Check sheet for the drawn part. Datum: minimum x, y, z corner. Units: mm. A direction names the side the tool comes from. Coordinates: 2 decimals unless noted, no trailing zeros. Loops run counter-clockwise (first coordinate to the right, second up) from the corner with the lowest first, then second, coordinate; pieces in that order, holes last.
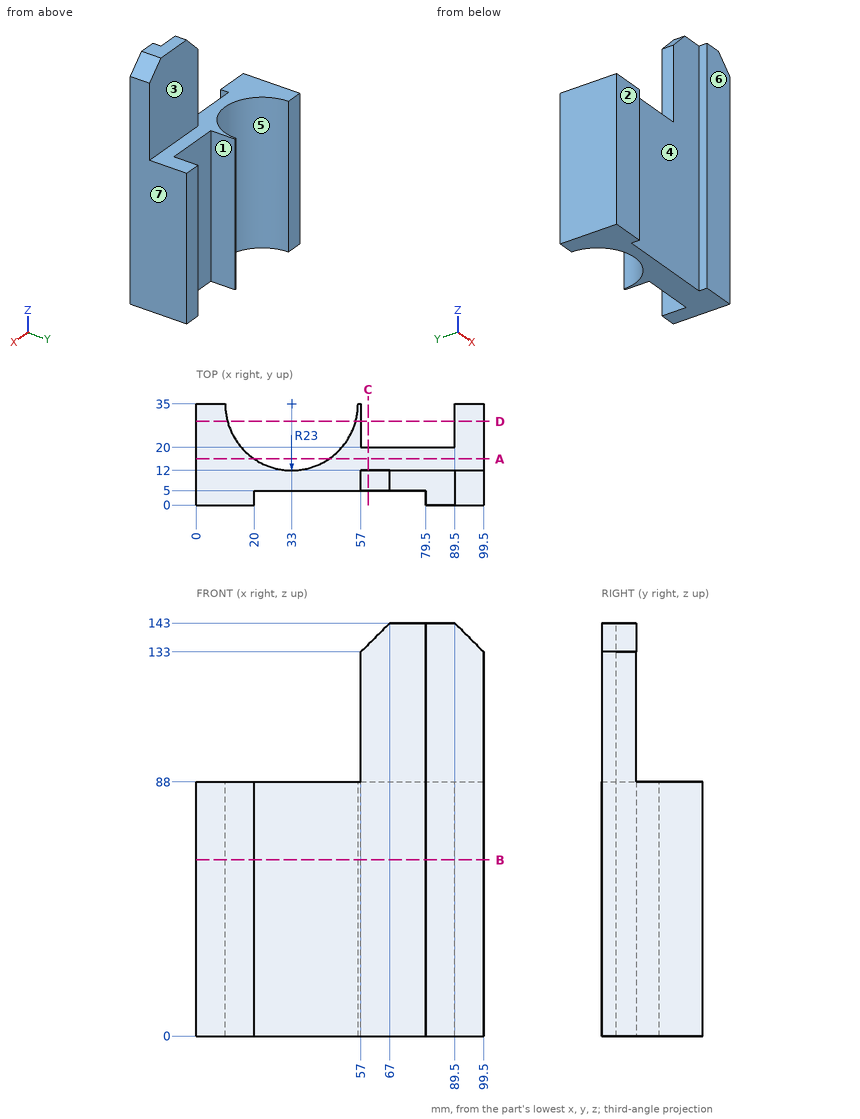
(1) Sectioned sample at A-A on y = 16. Record the cut outline in (x, z).
Findings:
outline: (0, 0) - (20.04, 0) - (20.04, 88) - (0, 88) - close; (45.96, 0) - (99.5, 0) - (99.5, 88) - (45.96, 88) - close
(2) Sectioned sample at B-B on z = 61. Record the cut outline in (x, y).
Findings:
outline: (0, 0) - (20, 0) - (20, 5) - (79.5, 5) - (79.5, 0) - (99.5, 0) - (99.5, 35) - (89.5, 35) - (89.5, 20) - (57, 20) - (57, 35) - (56, 35) arc R23 cw to (10, 35) - (0, 35) - close
(3) Sectioned sample at D-D on y = 29. Record the cut outline in (x, z), and give its area (3 significant figures).
Findings:
outline: (0, 0) - (10.8, 0) - (10.8, 88) - (0, 88) - close; (55.2, 0) - (57, 0) - (57, 88) - (55.2, 88) - close; (89.5, 0) - (99.5, 0) - (99.5, 88) - (89.5, 88) - close
area: 1,990 mm2
(4) Draft check along X on the marked faces 4, 5, 6 and 7. Enter one of: +X half, -X half, draft (parallel to the pull), parting line (faces both ways), or undercut.
Findings:
face 4: undercut
face 5: undercut
face 6: draft
face 7: +X half
(5) Sectioned sample at C-C on x = 59.5. Record the cut outline in (y, z), and give its area (3 significant figures).
Findings:
outline: (5, 0) - (20, 0) - (20, 88) - (12, 88) - (12, 135.5) - (5, 135.5) - close
area: 1,650 mm2
(6) Scan lines: L1, parallel to X at y = 21, z = 23.5; L2, parallel to Z at x = 24, y = 9; L3, parallel to X at y = 6, z = 89. Record each from-to range of solid material in increasing order.
Findings:
L1: x = 0 to 14.75, 51.25 to 57, 89.5 to 99.5
L2: z = 0 to 88
L3: x = 57 to 99.5
(7) Access from +Z, -Z, +X, -X, +Y, -Y to the whole of each face (thin tool, end or side, straight path). Record for the marked faces 1, 2 and 3.
Findings:
face 1: +Z, -Z, +Y
face 2: +Z, -Z, +X, -X, -Y
face 3: +Z, +X, -X, +Y
(8) Gauge pin test, flat ends, axial feed: pin 1 Ø8 at (y, z) = (4.5, 99.5) entering from -X; pin 2 Ø2 at (x, y) = (41, 15) entering from +Z; pin 3 Ø21 at (x, z) = (73.5, 114) entering from +Y; pin 4 Ø1 at (x, z) = (79.5, 22) entering from +Y. Record the tip position at first contact, or that the pin passes through.
Findings:
pin 1: stops at x = 57
pin 2: passes through
pin 3: stops at y = 12
pin 4: stops at y = 20
